The listing builds one solid part. Answer for the finished solid, in the listing's coordinates (mm). A direction names the side the tool comes from. Round coordinates to 2 decimals unless told otherwise and drop trailing zeros. Loops run counter-clockwise (first coordinate to the right, second up) from the corner with the lowest first, then second, coordinate; pieces in that order, holes last. Notation, with made-up numbers: M 3.25,80 L 14.25,80 A31 ccw 14.25,116 Z; hole C -39.75,21 d1. An arc over 180 degrees is marked long. Answer as a JSON object with one key per item and string values.
Autodesk Inventor part; units mm, degrees
ref_plane "YZ Plane" through (0, 0, 0) normal (1, 0, 0) x (0, 1, 0)
ref_plane "XZ Plane" through (0, 0, 0) normal (0, 1, 0) x (-1, 0, 0)
ref_plane "XY Plane" through (0, 0, 0) normal (0, 0, 1) x (1, 0, 0)
sketch "Sketch1" plane through (0, 0, 0) normal (0, 0, 1) x (1, 0, 0)
  circle A0 centre (0, 0) radius 8.4667
  circle A1 centre (0, 0) radius 12.7
  dimension "d4" = 25.4
extrude "Extrusion1" add sketch "Sketch1" along normal blind 127
sketch "Sketch2" plane through (0, 0, 0) normal (1, 0, 0) x (0, 1, 0)
  line L0 (-15.1143, 93.7374) -> (-1.5875, 93.7374)
  line L1 (-1.5875, 93.7374) -> (-1.5875, 33.1667)
  line L2 (-1.5875, 33.1667) -> (-15.1143, 33.1667)
  line L3 (-15.1143, 33.1667) -> (-15.1143, 93.7374)
  point P0 (0, 0)
extrude "Extrusion2" cut sketch "Sketch2" along normal mid plane 76.2
properties part number "WireCounterPiece2"
Item 1: Straight lines are drawn through the part: line 1 (Y direction, x = 1.5, z = 121); line 2 (Z direction, x = -6.5, y = -6.5); line 3 (Y direction, x = 0, z = 101). For each, find the intervals that lie inside material, in ascending order.
Values follow:
{"line 1": "-12.61 to -8.33, 8.33 to 12.61", "line 2": "0 to 33.17, 93.74 to 127", "line 3": "-12.7 to -8.47, 8.47 to 12.7"}
Item 2: The part is cut by section C-C (z = 26.5). Give the vertices of the cut face in (x, y), then the cut area to 3 significant figures.
Values follow:
{"outline": "C 0,0 d25.4; hole C 0,0 d16.93", "area": "282 mm^2"}
Item 3: The part is cut by section B-B (x = 0). Give the vertices of the cut face in (y, z), then the cut area to 3 significant figures.
Values follow:
{"outline": "M -12.7,0 L -8.47,0 L -8.47,33.17 L -12.7,33.17 Z; M -12.7,93.74 L -8.47,93.74 L -8.47,127 L -12.7,127 Z; M 8.47,0 L 12.7,0 L 12.7,127 L 8.47,127 Z", "area": "819 mm^2"}
Item 4: The part is cut by section D-D (y = -9.75). Give the vertices of the cut face in (x, z).
Values follow:
{"outline": "M -8.14,0 L 8.14,0 L 8.14,33.17 L -8.14,33.17 Z; M -8.14,93.74 L 8.14,93.74 L 8.14,127 L -8.14,127 Z"}
Item 5: Which of the six approach directions +Z, -Z, +X, -X, +Y, -Y give full straight-line access (tool end or side, diameter ignored) to faces 4 (the face through (0, -10, 33.167)), 5 (the face through (2.6, -8.3, 0))?
Values follow:
{"face 4": "+X, -X, -Y", "face 5": "-Z, +X, -X, +Y, -Y"}
Item 6: Flat-ended cylindrical pins translate along their axes: P1, Ø5, axis at x = 9, z = 25, coming from the +Y side; P2, Ø1.3, axis at x = 10, z = 74, coming from the -Y side; P3, Ø4, axis at x = 0.5, z = 69, coming from the -Y side. Find the tip coordinate at first contact, or state that the pin passes through.
Values follow:
{"P1": "y = 10.91", "P2": "y = -1.59", "P3": "y = 8.09"}
Item 7: The part is cut by section A-A (y = 0). Give the vertices of the cut face in (x, z).
Values follow:
{"outline": "M -12.7,0 L -8.47,0 L -8.47,127 L -12.7,127 Z; M 8.47,0 L 12.7,0 L 12.7,127 L 8.47,127 Z"}
Item 8: Determine the mould class of faces 1 (the face through (-1.835, 8.265, 62.611)), 2 (the face through (2.6, -8.3, 127)), 3 (the face through (-10, -1.588, 64)) for opening direction Y: released by +Y, released by -Y, zero draft, split by the parting line, or undercut.
Values follow:
{"face 1": "undercut", "face 2": "zero draft", "face 3": "released by -Y"}
